Build history of the part. All positions in model axes, mm. Round coordinates to 2 decimals unless told otherwise and drop trailing zeros. Order: outer loops, then holes, each group sorted by start corner. A loop starts at its lowest first (then second) coordinate and runs counter-clockwise, first axis right, second up. Notation, with made-up numbers: M 35.25,-14 L 92.25,-14 A17 cw 92.25,15 Z; hole C 19,70.5 d8. An arc over 180 degrees is marked long. One line per item, written item: value. Start each with the question number.
Item 1: Pin check, flat tips, straight feed: pin 1 (4.5 mm diameter, centred on x = -135, y = 943, fed in from +Z); pin 2 (0.9 mm diameter, centred on x = -289.5, z = 1.5, fed in from +Y). Stop position of each tip, or through.
Item 2: Band-saw the part on A-A, the plane z = 0.45. Write the cut outline in (x, y).
Item 3: Probe L1, parallel to X at y = 1090, z = 2.25; L2, parallel to Y at x = -135, z = 1.2; L3, parallel to Y at x = -355, z = 1.9. List the from-to ranges inside material, lowest first.
```python
from build123d import *

# Parameters (mm, degrees)
BOX002_W          = 32
BOX002_H          = 62
BOX002_DEPTH      = 9
CYLINDER_R        = 2.5
CYLINDER_DEPTH    = 10
CYLINDER001_R     = 2.5
CYLINDER001_DEPTH = 100
CYLINDER002_R     = 2.5
CYLINDER002_DEPTH = 100
CYLINDER003_R     = 2.5
CYLINDER003_DEPTH = 100
CYLINDER004_R     = 2.5
CYLINDER004_DEPTH = 100
BOX001_W          = 62
BOX001_H          = 32
BOX001_DEPTH      = 9
BOX_W             = 440
BOX_H             = 310
BOX_DEPTH         = 3


with BuildPart() as electronics_base002:
    # Box002 → Box002 (new body)
    with BuildSketch(Plane(origin=(-151, 785, -1), x_dir=(1, 0, 0), z_dir=(0, 0, 1))):
        with Locations((16, 31)):
            Rectangle(BOX002_W, BOX002_H)
    extrude(amount=BOX002_DEPTH)


with BuildPart() as cylinder:
    # Cylinder → Cylinder (new body)
    with BuildSketch(Plane(origin=(64, 1090, -3), x_dir=(1, 0, 0), z_dir=(0, 0, 1))):
        Circle(CYLINDER_R)
    extrude(amount=CYLINDER_DEPTH)


with BuildPart() as cylinder001:
    # Cylinder001 → Cylinder001 (new body)
    with BuildSketch(Plane(origin=(-135, 1090, -45), x_dir=(1, 0, 0), z_dir=(0, 0, 1))):
        Circle(CYLINDER001_R)
    extrude(amount=CYLINDER001_DEPTH)


with BuildPart() as cylinder002:
    # Cylinder002 → Cylinder002 (new body)
    with BuildSketch(Plane(origin=(-355, 1090, -45), x_dir=(1, 0, 0), z_dir=(0, 0, 1))):
        Circle(CYLINDER002_R)
    extrude(amount=CYLINDER002_DEPTH)


with BuildPart() as cylinder003:
    # Cylinder003 → Cylinder003 (new body)
    with BuildSketch(Plane(origin=(-355, 810, -45), x_dir=(1, 0, 0), z_dir=(0, 0, 1))):
        Circle(CYLINDER003_R)
    extrude(amount=CYLINDER003_DEPTH)


with BuildPart() as cylinder004:
    # Cylinder004 → Cylinder004 (new body)
    with BuildSketch(Plane(origin=(-135, 943, -45), x_dir=(1, 0, 0), z_dir=(0, 0, 1))):
        Circle(CYLINDER004_R)
    extrude(amount=CYLINDER004_DEPTH)


with BuildPart() as cuts_electronic_base:
    # Box001 → Box001 (new body)
    with BuildSketch(Plane(origin=(-312, 1074, -1), x_dir=(1, 0, 0), z_dir=(0, 0, 1))):
        with Locations((31, 16)):
            Rectangle(BOX001_W, BOX001_H)
    extrude(amount=BOX001_DEPTH)

    # Fusion001002: union electronics_base002, Cylinder, Cylinder001, Cylinder002, Cylinder003, Cylinder004
    add(electronics_base002.part)
    add(cylinder.part)
    add(cylinder001.part)
    add(cylinder002.part)
    add(cylinder003.part)
    add(cylinder004.part)


with BuildPart() as wood_electronic_base:
    # Box → Box (new body)
    with BuildSketch(Plane(origin=(-370, 795, 0), x_dir=(1, 0, 0), z_dir=(0, 0, 1))):
        with Locations((220, 155)):
            Rectangle(BOX_W, BOX_H)
    extrude(amount=BOX_DEPTH)

    # Cut: cut cuts_electronic_base
    add(cuts_electronic_base.part, mode=Mode.SUBTRACT)


solid = wood_electronic_base.part
```
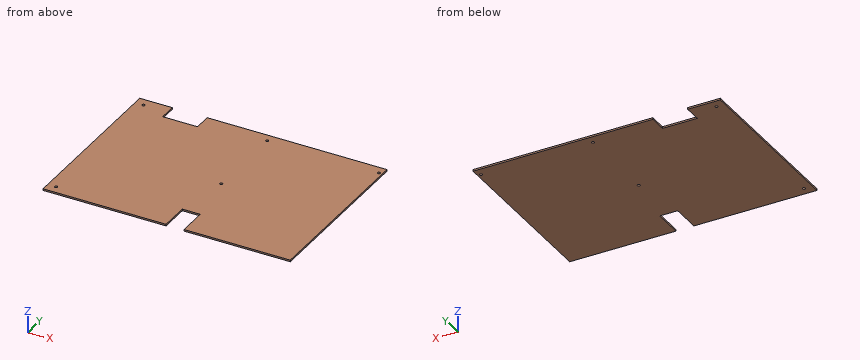
Output:
1. pin 1: passes through
1. pin 2: stops at y = 1074
2. outline: M -370,795 L -151,795 L -151,847 L -119,847 L -119,795 L 70,795 L 70,1105 L -250,1105 L -250,1074 L -312,1074 L -312,1105 L -370,1105 Z; hole C -355,810 d5; hole C -355,1090 d5; hole C -135,943 d5; hole C -135,1090 d5; hole C 64,1090 d5
3. L1: x = -370 to -357.5, -352.5 to -312, -250 to -137.5, -132.5 to 61.5, 66.5 to 70
3. L2: y = 847 to 940.5, 945.5 to 1087.5, 1092.5 to 1105
3. L3: y = 795 to 807.5, 812.5 to 1087.5, 1092.5 to 1105
